Check sheet for the drawn part. Datum: minimum x, y, z corner. Units: mm. Give positions to 0.01 mm unless a question says otherwise; leave off trailing zeros. Order: outer loops, then holes, each group sorted by start corner. A loop starts at its lowest first (then second) coordinate and runs counter-clockwise, first axis right, second up.
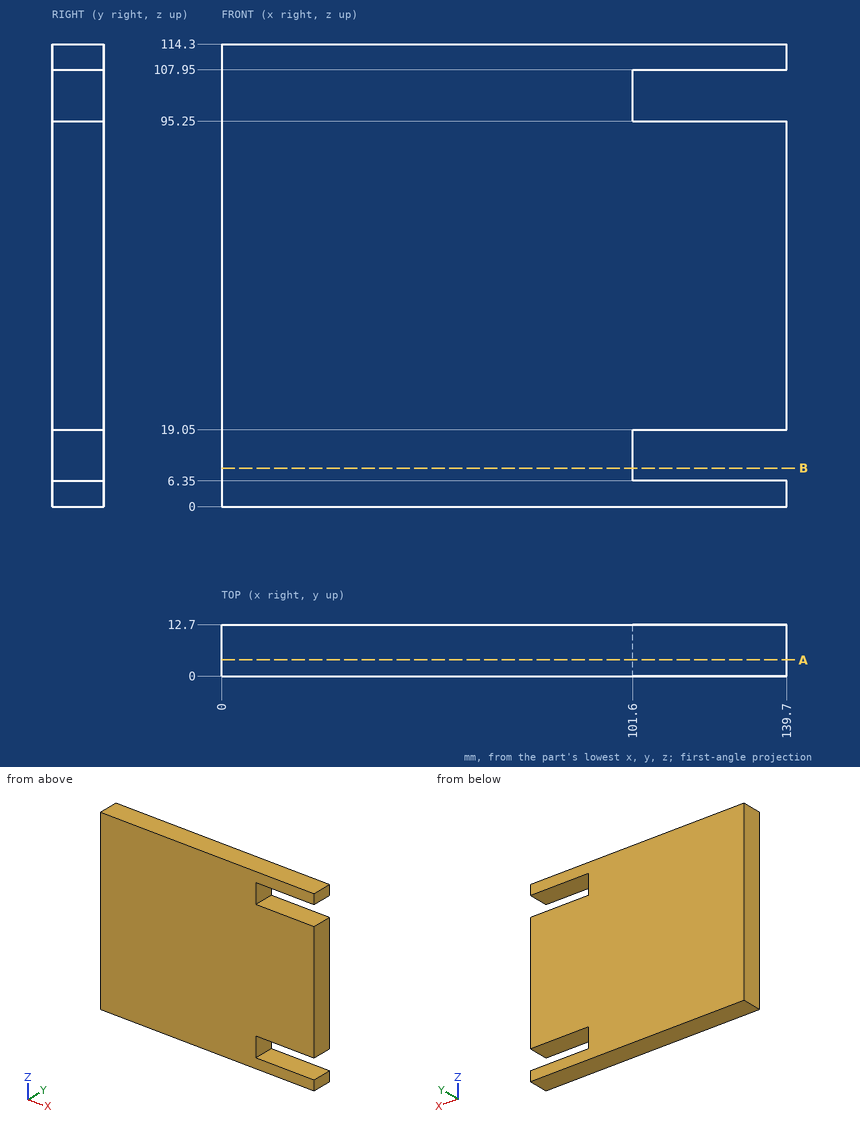
Item 1: Scan lines: L1, parallel to Z at x = 123.5, y = 5.5; L2, parallel to X at y = 8.75, z = 13. Record each from-to range of solid material in increasing order.
Reported:
L1: z = 0 to 6.35, 19.05 to 95.25, 107.95 to 114.3
L2: x = 0 to 101.6
Item 2: Gauge pin test, flat end, axial feed: pin 1 (3 mm diameter, centred on y = 3, z = 15, fed in from +X). Record the tip position at first contact, or that the pin passes through.
Reported:
pin 1: stops at x = 101.6
Item 3: Sectioned sample at A-A (y = 4). Enter the section's corners in (x, z), and give its area (3 significant figures).
Reported:
outline: (0, 0) - (139.7, 0) - (139.7, 6.35) - (101.6, 6.35) - (101.6, 19.05) - (139.7, 19.05) - (139.7, 95.25) - (101.6, 95.25) - (101.6, 107.95) - (139.7, 107.95) - (139.7, 114.3) - (0, 114.3) - close
area: 15,000 mm2
Item 4: Sectioned sample at B-B (z = 9.5). Enter the section's corners in (x, y).
Reported:
outline: (0, 0) - (101.6, 0) - (101.6, 12.7) - (0, 12.7) - close
